```python
from build123d import *

# Parameters (mm, degrees)
SKETCH_1_R          = 3.525
EXTRUDE_1_DEPTH     = 4
FILLET_1_R          = 10
CHAMFER_1_SIZE      = 0.5
SKETCH_3_R          = 4.125
CUT_EXTRUDE_2_DEPTH = 0.1
CUT_EXTRUDE_START   = -0.1
SKETCH_4_R          = 4.125
CUT_EXTRUDE_3_DEPTH = 0.1


with BuildPart() as part:
    # 草图1 → 凸台-拉伸1 (new body)
    with BuildSketch(Plane(origin=(0, 0, 0), x_dir=(1, 0, 0), z_dir=(0, 1, 0))):
        with BuildLine():
            Line((4.898979486, 2.5), (115.101020514, 2.5))
            ThreePointArc((115.101020514, 2.5), (125.5, 0), (115.101020514, -2.5))
            Line((115.101020514, -2.5), (4.898979486, -2.5))
            ThreePointArc((4.898979486, -2.5), (-5.5, 0), (4.898979486, 2.5))
        make_face()
        with Locations(Location((0, 0, 0), (0, 0, 270))):
            Circle(SKETCH_1_R, mode=Mode.SUBTRACT)
        with Locations(Location((120, 0, 0), (0, 0, 270))):
            Circle(SKETCH_1_R, mode=Mode.SUBTRACT)
    extrude(amount=EXTRUDE_1_DEPTH)

    # 圆角1
    fillet_1_edges = [part.edges().sort_by_distance(p)[0] for p in [
        (4.898979486, 2, -2.5),
        (115.101020514, 2, -2.5),
        (115.101020514, 2, 2.5),
        (4.898979486, 2, 2.5),
    ]]
    fillet(fillet_1_edges, radius=FILLET_1_R)

    # 倒角1
    chamfer_1_edges = [part.edges().sort_by_distance(p)[0] for p in [
        (125.5, 0, 0),
        (125.5, 4, 0),
        (60, 0, 2.5),
        (60, 4, 2.5),
        (60, 0, -2.5),
        (60, 4, -2.5),
        (-5.5, 0, 0),
        (-5.5, 4, 0),
        (113.945703694, 0, 2.996180734),
        (113.945703694, 4, 2.996180734),
        (113.945703694, 0, -2.996180734),
        (113.945703694, 4, -2.996180734),
        (6.054296306, 0, 2.996180734),
        (6.054296306, 4, 2.996180734),
        (6.054296306, 0, -2.996180734),
        (6.054296306, 4, -2.996180734),
    ]]
    chamfer(chamfer_1_edges, length=CHAMFER_1_SIZE)

    # 草图3 → 切除-拉伸2 (cut)
    with BuildSketch(Plane(origin=(0, 4, 0), x_dir=(1, 0, 0), z_dir=(0, 1, 0))):
        with Locations(Location((0, 0, 0), (0, 0, 270))):
            Circle(SKETCH_3_R)
        with Locations(Location((120, 0, 0), (0, 0, 270))):
            Circle(SKETCH_3_R)
    extrude(amount=-CUT_EXTRUDE_2_DEPTH, mode=Mode.SUBTRACT)

    # 草图4 → 切除-拉伸3 (cut)
    with BuildSketch(Plane.XZ.offset(CUT_EXTRUDE_START)):
        with Locations(Location((0, 0, 0), (0, 0, 90))):
            Circle(SKETCH_4_R)
        with Locations(Location((120, 0, 0), (0, 0, 90))):
            Circle(SKETCH_4_R)
    extrude(amount=CUT_EXTRUDE_3_DEPTH, mode=Mode.SUBTRACT)


solid = part.part
```
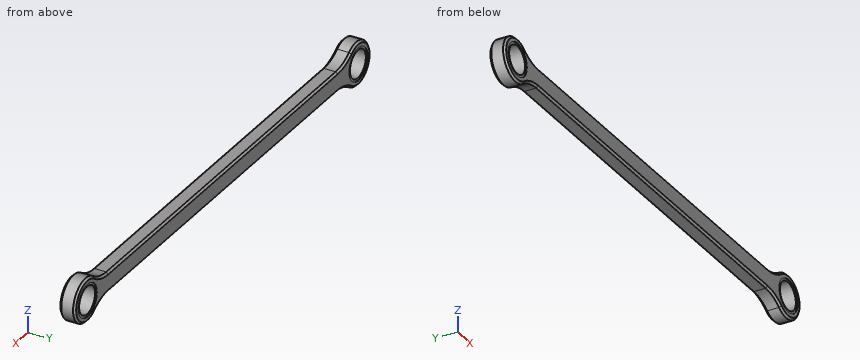
Part model, mm, in its own coordinate system. Round coordinates to 2 decimals unless told otherwise and drop trailing zeros. Order: outer loops, then holes, each group sorted by start corner. A loop starts at its lowest first (then second) coordinate and runs counter-clockwise, first axis right, second up. Notation, with made-up numbers: M 69.5,53 L 119.5,53 A28 cw 119.5,90 Z; hole C 25,26 d4. An arc over 180 degrees is marked long. Answer in a Markdown table with one row per item. Add a question column.
Q1. Wall check: L1, parallel to X at y = 2.9, z = 0 (3 decimals); L2, parallel to Z at x = 0, y = 1.25 (3 decimals); L3, parallel to X at y = 3.7, z = 2. Give the ranges that are in metal, low to high. Write a range as from..to.
Q2. Cut at B-B on y = 1.45. Give the cut face in (x, z) (3 decimals).
Q3. Cut at A-A on z = 0. Give the number of separate pieces and of enclosed holes in the cut face, and give its area (3 significant figures).
Q4. Cut at C-C on x = 120. Give the cut face in (y, z) (3 decimals), and give its area (3 significant figures).
Q5. Cut at D-D on x = 17.5. Give the cut face in (y, z).
Q6. Pin check, flat tip, straight feed: pin 1 (1.5 mm diameter, centred on y = 2.5, z = 2.5, fed in from +X). Stop position of the tip, or through.
Established:
| question | item | result |
|---|---|---|
| 1 | L1 | x = -5.5..-3.525, 3.525..116.475, 123.525..125.5 |
| 1 | L2 | z = -5.5..-3.525, 3.525..5.5 |
| 1 | L3 | x = -4.91..-2.9, 2.9..117.1, 122.9..124.91 |
| 2 | outline | M 3.252,-4.435 A10 cw 9.165,-2.5 L 110.835,-2.5 A10 cw 116.748,-4.435 A5.5 ccw long 116.748,4.435 A10 cw 110.835,2.5 L 9.165,2.5 A10 cw 3.252,4.435 A5.5 ccw long Z; hole C 0,0 d7.05; hole C 120,0 d7.05 |
| 3 | separate pieces | 3 |
| 3 | enclosed holes | 0 |
| 3 | area | 467 mm2 |
| 4 | outline | M 0,-5 L 0.5,-5.5 L 3.5,-5.5 L 4,-5 L 4,-4.125 L 3.9,-4.125 L 3.9,-3.525 L 0.1,-3.525 L 0.1,-4.125 L 0,-4.125 Z; M 0,4.125 L 0.1,4.125 L 0.1,3.525 L 3.9,3.525 L 3.9,4.125 L 4,4.125 L 4,5 L 3.5,5.5 L 0.5,5.5 L 0,5 Z |
| 4 | area | 15.1 mm2 |
| 5 | outline | M 0,-2 L 0.5,-2.5 L 3.5,-2.5 L 4,-2 L 4,2 L 3.5,2.5 L 0.5,2.5 L 0,2 Z |
| 6 | pin 1 | stops at x = 125.21 |
